The model under review builds one solid part; all positions refer to its coordinate system, in mm. A direction names the side the tool comes from. Give positions to 0.01 mm unless a question says otherwise; leave off trailing zeros. Order: outer loops, then holes, each group sorted by start corner. A loop starts at its lowest first (then second) coordinate and runs counter-clockwise, first axis right, second up. Notation, with made-up numbers: (22, 26) - (56, 26) arc R31 cw to (56, 59) - close; hole circle Ø10 at (-30, -30.5). An arc over 180 degrees is marked (long way). Use a Markdown table: item, result. Add a question column.
```python
from build123d import *


with BuildPart() as part:
    # Sketch1 → Revolve1 (revolve)
    with BuildSketch(Plane.XY, mode=Mode.PRIVATE) as revolve1_sk:
        with BuildLine():
            Line((0, 5.9), (0, 14))
            Line((0, 14), (3, 14))
            Line((3, 14), (3, 8.2))
            ThreePointArc((3, 8.2), (3.439339828, 7.139339828), (4.5, 6.7))
            Line((4.5, 6.7), (41.5, 6.7))
            ThreePointArc((41.5, 6.7), (42.560660172, 7.139339828), (43, 8.2))
            Line((43, 8.2), (43, 14))
            Line((43, 14), (46, 14))
            Line((46, 14), (46, 5.9))
            Line((46, 5.9), (43, 5.9))
            Line((43, 5.9), (3, 5.9))
            Line((3, 5.9), (0, 5.9))
        make_face()
    revolve(revolve1_sk.sketch.rotate(Axis((0, 0, 0), (-1, 0, 0)), 90), axis=Axis((0, 0, 0), (-1, 0, 0)))


solid = part.part
```
Q1. We need section D-D (z = -8.75). Write out the cut boundary in (x, y), plus the area to 3 significant figures.
Q2. Wall thickness on probe 1 along X at (y, z) = (9, -9.5); probe 2 along Y at (x, z) = (27, 0); probe 3 along Y at (x, z) = (42, -2.5): over which ranges is each line inside the solid? List them lowest first.
Q3. Machinability: for faces 4 (the flat face through (46, 6, -3)), 5 (the flat face through (3, 6, -6)), which of the approach directions +Z, -Z, +X, -X, +Y, -Y give a long, thin tool a straight path to every point of the face, cutting with its end or side? Answer none if there is none.
Q4. Draft analysis for pull direction X (two halves, no side actions). For faces 1 (the flat face through (0, 6, 3)), 2 (the flat face through (43, 6, 6)), 3 (the cylindrical face through (22.678, -0.259, 5.894)), state which applies: pulls with the +X half, pulls with the -X half, needs draft (parallel to the pull), parting line crosses it, or undercut.
Q5. We need section A-A (y = 0). Write out the cut boundary in (x, z).
Q6. Clearance check with flat-ended pins moving along their axes: P1, Ø4, axis at x = 11, z = 3.5, coming from the -Y side; P2, Ø1, axis at x = 22.5, y = -6.5, coming from the +Z side; P3, Ø10, axis at x = 28, y = 9, coming from the -Z side. State where each tip first meets the part, or that it passes through.
Q7. We need section C-C (x = 13). Write out the cut boundary in (y, z), plus the area to 3 significant figures.
Here are the results:
| question | item | result |
|---|---|---|
| 1 | outline | (0, -10.93) - (3, -10.93) - (3, 10.93) - (0, 10.93) - close; (43, -10.93) - (46, -10.93) - (46, 10.93) - (43, 10.93) - close |
| 1 | area | 131 mm2 |
| 2 | probe 1 | 0 to 3, 43 to 46 |
| 2 | probe 2 | -6.7 to -5.9, 5.9 to 6.7 |
| 2 | probe 3 | -6.31 to -5.34, 5.34 to 6.31 |
| 3 | face 4 | +Z, -Z, +X, +Y, -Y |
| 3 | face 5 | none |
| 4 | face 1 | pulls with the -X half |
| 4 | face 2 | undercut |
| 4 | face 3 | needs draft |
| 5 | outline | (0, -14) - (3, -14) - (3, -8.2) arc R1.5 cw to (4.5, -6.7) - (41.5, -6.7) arc R1.5 cw to (43, -8.2) - (43, -14) - (46, -14) - (46, -5.9) - (0, -5.9) - close; (0, 5.9) - (46, 5.9) - (46, 14) - (43, 14) - (43, 8.2) arc R1.5 cw to (41.5, 6.7) - (4.5, 6.7) arc R1.5 cw to (3, 8.2) - (3, 14) - (0, 14) - close |
| 6 | P1 | y = -6.53 |
| 6 | P2 | z = 2.98 |
| 6 | P3 | z = -5.37 |
| 7 | outline | circle Ø13.4 at (0, 0); hole circle Ø11.8 at (0, 0) |
| 7 | area | 31.7 mm2 |
